Geometry check sheet. Reference: drawing and pictorial views, mm from the part's lowest x, y, z. A direction names the side the tool comes from. Give positions to 0.01 mm unless a question says otherwise; leave off trailing zeros. Write each loop counter-clockwise with the first axis right and the second up, starting at its lowest first coordinate (ties: lowest second). Pieces come first, ordered by that corner, then holes. Notation, with made-up numbers: M -22,-2.5 L 13,-2.5 A13 ccw 13,2.5 Z; hole C -32,30 d10. An arc over 180 degrees is marked long. Write item = value, one per line. Start each with the question number.
1) Mould release check, pull along Y, two halves, no side actions. Record for the marked faces 5, 6, 7 and 8: released by +Y, released by -Y, zero draft, split by the parting line, or undercut.
2) Cross-section at D-D, the plane x = 9. Record the cut outline in (y, z) (1 decimal).
3) Cross-section at A-A, the plane y = 8. Record the cut outline in (x, z).
4) Access from +Z, -Z, +X, -X, +Y, -Y to the whole of each face (thin tool, end or side, straight path). Record for the marked faces 1, 2, 3 and 4.
5) Scan lines: line 1 along Y through (x, z) = (23.5, 5.5); line 2 along X through (y, z) = (7, 5.5); line 3 along X through (y, z) = (14, 2.5). Record each from-to range of solid material in increasing order. Write a range as [from, to].
6) Cross-section at C-C, the plane x = 17.5. Record the cut outline in (y, z), plus the area to 3 significant figures.
7) Cross-section at B-B, the plane z = 13.75. Record the cut outline in (x, y) (1 decimal).
8) Go/stop test with flat-tipped pins: pin 1 (4.5 mm diameter, centred on y = 8.5, z = 5.5, fed in from +X); pin 2 (10 mm diameter, centred on y = 10, z = 10.5, fed in from -X); pin 3 (12 mm diameter, centred on y = 14.5, z = 7.5, fed in from -X). Record where each tip stops, or that it passes through.
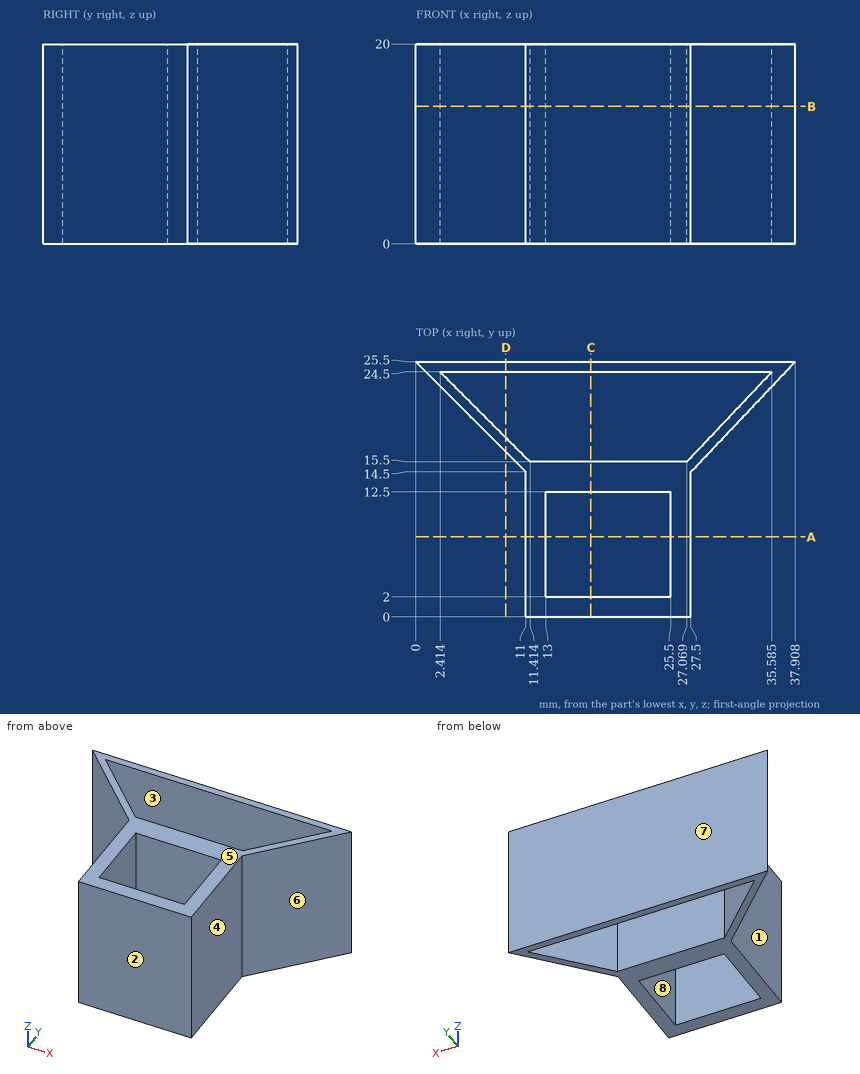
Reply:
q1.face_5 = zero draft
q1.face_6 = released by -Y
q1.face_7 = released by +Y
q1.face_8 = undercut
q2.outline = M 16.5,0 L 17.9,0 L 17.9,20 L 16.5,20 Z; M 24.5,0 L 25.5,0 L 25.5,20 L 24.5,20 Z
q3.outline = M 11,0 L 13,0 L 13,20 L 11,20 Z; M 25.5,0 L 27.5,0 L 27.5,20 L 25.5,20 Z
q4.face_1 = +Z, -Z, -X, -Y
q4.face_2 = +Z, -Z, +X, -X, -Y
q4.face_3 = +Z, -Z
q4.face_4 = +Z, -Z, +X, -Y
q5.line_1 = [0, 2], [12.5, 15.5], [24.5, 25.5]
q5.line_2 = [11, 13], [25.5, 27.5]
q5.line_3 = [11, 27.5]
q6.outline = M 0,0 L 2,0 L 2,20 L 0,20 Z; M 12.5,0 L 15.5,0 L 15.5,20 L 12.5,20 Z; M 24.5,0 L 25.5,0 L 25.5,20 L 24.5,20 Z
q6.area = 120 mm2
q7.outline = M 0,25.5 L 11,14.5 L 11,0 L 27.5,0 L 27.5,14.5 L 37.9,25.5 Z; hole M 2.4,24.5 L 11.4,15.5 L 27.1,15.5 L 35.6,24.5 Z; hole M 13,2 L 25.5,2 L 25.5,12.5 L 13,12.5 Z
q8.pin_1 = 27.5
q8.pin_2 = 10.5
q8.pin_3 = 5
